Verification items for the finished model (mm, model axes). Face numbers are marked on the shaded views. A direction names the side the tool comes from. Round coordinates to 2 decimals unless told otherwise and drop trailing zeros. One line per item, written item: value. Start each with the question number.
from build123d import *

# Parameters (mm, degrees)
SKETCH1_R           = 8.345
SKETCH1_R_2         = 7.045
BOSS_EXTRUDE1_DEPTH = 7.92
SKETCH2_R           = 7.045000007
BOSS_EXTRUDE2_DEPTH = 1.02
BOSS_EXTRUDE3_REACH = 9.92
BOSS_EXTRUDE4_DEPTH = 0.51
SKETCH5_W           = 1.28
SKETCH5_H           = 2.28
SKETCH5_W_2         = 2.28
SKETCH5_H_2         = 1.28
BOSS_EXTRUDE5_DEPTH = 2.41
CUT_EXTRUDE1_DEPTH  = 9.985
CUT_EXTRUDE2_DEPTH  = 2.41
CUT_EXTRUDE3_DEPTH  = 2.41


with BuildPart() as part:
    # Sketch1 → Boss-Extrude1 (new body)
    with BuildSketch(Plane(origin=(0, 0, 0), x_dir=(1, 0, 0), z_dir=(0, 1, 0))):
        Circle(SKETCH1_R)
        Circle(SKETCH1_R_2, mode=Mode.SUBTRACT)
    extrude(amount=BOSS_EXTRUDE1_DEPTH)

    # Sketch2 → Boss-Extrude2 (add)
    with BuildSketch(Plane(origin=(0, 0, 0), x_dir=(1, 0, 0), z_dir=(0, 1, 0))):
        Circle(SKETCH2_R)
    extrude(amount=BOSS_EXTRUDE2_DEPTH)

    # Sketch3 → Boss-Extrude3 (add, up to next)
    with BuildSketch(Plane(origin=(0, 7.92, 0), x_dir=(1, 0, 0), z_dir=(0, 1, 0)), mode=Mode.PRIVATE) as boss_extrude3_sk1:
        with BuildLine():
            Line((-0.455000106, 4.724999874), (0.455000106, 4.724999874))
            Line((0.455000106, 4.724999874), (0.455000106, 8.332586627))
            ThreePointArc((0.455000106, 8.332586627), (0, 8.345), (-0.455000106, 8.332586627))
            Line((-0.455000106, 8.332586627), (-0.455000106, 4.724999874))
        make_face()
    boss_extrude3_tool1 = extrude(boss_extrude3_sk1.sketch, amount=-BOSS_EXTRUDE3_REACH, mode=Mode.PRIVATE) - part.part
    add(boss_extrude3_tool1.solids().sort_by_distance((0, 7.92, -6.532934))[0])
    # Sketch3 → Boss-Extrude3 (add, up to next)
    with BuildSketch(Plane(origin=(0, 7.92, 0), x_dir=(1, 0, 0), z_dir=(0, 1, 0)), mode=Mode.PRIVATE) as boss_extrude3_sk2:
        with BuildLine():
            Line((3.019345792, 3.662813112), (5.570294849, 6.213762169))
            ThreePointArc((5.570294849, 6.213762169), (5.900806089, 5.900806089), (6.213762169, 5.570294849))
            Line((6.213762169, 5.570294849), (3.662813112, 3.019345792))
            Line((3.662813112, 3.019345792), (3.019345792, 3.662813112))
        make_face()
    boss_extrude3_tool2 = extrude(boss_extrude3_sk2.sketch, amount=-BOSS_EXTRUDE3_REACH, mode=Mode.PRIVATE) - part.part
    add(boss_extrude3_tool2.solids().sort_by_distance((4.619482, 7.92, -4.619482))[0])
    # Sketch3 → Boss-Extrude3 (add, up to next)
    with BuildSketch(Plane(origin=(0, 7.92, 0), x_dir=(1, 0, 0), z_dir=(0, 1, 0)), mode=Mode.PRIVATE) as boss_extrude3_sk3:
        with BuildLine():
            Line((4.724999874, 0.455000106), (8.332586627, 0.455000106))
            ThreePointArc((8.332586627, 0.455000106), (8.345, 0), (8.332586627, -0.455000106))
            Line((8.332586627, -0.455000106), (4.724999874, -0.455000106))
            Line((4.724999874, -0.455000106), (4.724999874, 0.455000106))
        make_face()
    boss_extrude3_tool3 = extrude(boss_extrude3_sk3.sketch, amount=-BOSS_EXTRUDE3_REACH, mode=Mode.PRIVATE) - part.part
    add(boss_extrude3_tool3.solids().sort_by_distance((6.532934, 7.92, 0))[0])
    # Sketch3 → Boss-Extrude3 (add, up to next)
    with BuildSketch(Plane(origin=(0, 7.92, 0), x_dir=(1, 0, 0), z_dir=(0, 1, 0)), mode=Mode.PRIVATE) as boss_extrude3_sk4:
        with BuildLine():
            Line((3.662813112, -3.019345792), (6.213762169, -5.570294849))
            ThreePointArc((6.213762169, -5.570294849), (5.900806089, -5.900806089), (5.570294849, -6.213762169))
            Line((5.570294849, -6.213762169), (3.019345792, -3.662813112))
            Line((3.019345792, -3.662813112), (3.662813112, -3.019345792))
        make_face()
    boss_extrude3_tool4 = extrude(boss_extrude3_sk4.sketch, amount=-BOSS_EXTRUDE3_REACH, mode=Mode.PRIVATE) - part.part
    add(boss_extrude3_tool4.solids().sort_by_distance((4.619482, 7.92, 4.619482))[0])
    # Sketch3 → Boss-Extrude3 (add, up to next)
    with BuildSketch(Plane(origin=(0, 7.92, 0), x_dir=(1, 0, 0), z_dir=(0, 1, 0)), mode=Mode.PRIVATE) as boss_extrude3_sk5:
        with BuildLine():
            Line((0.455000106, -4.724999874), (0.455000106, -8.332586627))
            ThreePointArc((0.455000106, -8.332586627), (0, -8.345), (-0.455000106, -8.332586627))
            Line((-0.455000106, -8.332586627), (-0.455000106, -4.724999874))
            Line((-0.455000106, -4.724999874), (0.455000106, -4.724999874))
        make_face()
    boss_extrude3_tool5 = extrude(boss_extrude3_sk5.sketch, amount=-BOSS_EXTRUDE3_REACH, mode=Mode.PRIVATE) - part.part
    add(boss_extrude3_tool5.solids().sort_by_distance((0, 7.92, 6.532934))[0])
    # Sketch3 → Boss-Extrude3 (add, up to next)
    with BuildSketch(Plane(origin=(0, 7.92, 0), x_dir=(1, 0, 0), z_dir=(0, 1, 0)), mode=Mode.PRIVATE) as boss_extrude3_sk6:
        with BuildLine():
            Line((-3.019345792, -3.662813112), (-5.570294849, -6.213762169))
            ThreePointArc((-5.570294849, -6.213762169), (-5.900806089, -5.900806089), (-6.213762169, -5.570294849))
            Line((-6.213762169, -5.570294849), (-3.662813112, -3.019345792))
            Line((-3.662813112, -3.019345792), (-3.019345792, -3.662813112))
        make_face()
    boss_extrude3_tool6 = extrude(boss_extrude3_sk6.sketch, amount=-BOSS_EXTRUDE3_REACH, mode=Mode.PRIVATE) - part.part
    add(boss_extrude3_tool6.solids().sort_by_distance((-4.619482, 7.92, 4.619482))[0])
    # Sketch3 → Boss-Extrude3 (add, up to next)
    with BuildSketch(Plane(origin=(0, 7.92, 0), x_dir=(1, 0, 0), z_dir=(0, 1, 0)), mode=Mode.PRIVATE) as boss_extrude3_sk7:
        with BuildLine():
            Line((-4.724999874, -0.455000106), (-8.332586627, -0.455000106))
            ThreePointArc((-8.332586627, -0.455000106), (-8.345, 0), (-8.332586627, 0.455000106))
            Line((-8.332586627, 0.455000106), (-4.724999874, 0.455000106))
            Line((-4.724999874, 0.455000106), (-4.724999874, -0.455000106))
        make_face()
    boss_extrude3_tool7 = extrude(boss_extrude3_sk7.sketch, amount=-BOSS_EXTRUDE3_REACH, mode=Mode.PRIVATE) - part.part
    add(boss_extrude3_tool7.solids().sort_by_distance((-6.532934, 7.92, 0))[0])
    # Sketch3 → Boss-Extrude3 (add, up to next)
    with BuildSketch(Plane(origin=(0, 7.92, 0), x_dir=(1, 0, 0), z_dir=(0, 1, 0)), mode=Mode.PRIVATE) as boss_extrude3_sk8:
        with BuildLine():
            Line((-3.662813112, 3.019345792), (-6.213762169, 5.570294849))
            ThreePointArc((-6.213762169, 5.570294849), (-5.900806089, 5.900806089), (-5.570294849, 6.213762169))
            Line((-5.570294849, 6.213762169), (-3.019345792, 3.662813112))
            Line((-3.019345792, 3.662813112), (-3.662813112, 3.019345792))
        make_face()
    boss_extrude3_tool8 = extrude(boss_extrude3_sk8.sketch, amount=-BOSS_EXTRUDE3_REACH, mode=Mode.PRIVATE) - part.part
    add(boss_extrude3_tool8.solids().sort_by_distance((-4.619482, 7.92, -4.619482))[0])

    # Sketch4 → Boss-Extrude4 (add)
    with BuildSketch(Plane.XZ):
        with BuildLine():
            Line((-3.069700642, 2.308712987), (-6.179087875, 5.238791894))
            ThreePointArc((-6.179087875, 5.238791894), (-8.097423758, -0.240407921), (-5.857404636, -5.596148534))
            Line((-5.857404636, -5.596148534), (-2.927325729, -2.486761301))
            ThreePointArc((-2.927325729, -2.486761301), (-3.839300032, -0.113986642), (-3.069700642, 2.308712987))
        make_face()
        with BuildLine():
            Line((2.308712987, 3.069700642), (5.238791894, 6.179087875))
            ThreePointArc((5.238791894, 6.179087875), (-0.240407921, 8.097423758), (-5.596148534, 5.857404636))
            Line((-5.596148534, 5.857404636), (-2.486761301, 2.927325729))
            ThreePointArc((-2.486761301, 2.927325729), (-0.113986642, 3.839300032), (2.308712987, 3.069700642))
        make_face()
        with BuildLine():
            ThreePointArc((8.100991759, 0), (7.519203886, 3.014571346), (5.857404636, 5.596148534))
            Line((5.857404636, 5.596148534), (2.927325729, 2.486761301))
            ThreePointArc((2.927325729, 2.486761301), (3.605346841, 1.324647819), (3.840991759, 0))
            ThreePointArc((3.840991759, 0), (3.643069623, -1.217070832), (3.069700642, -2.308712987))
            Line((3.069700642, -2.308712987), (6.179087875, -5.238791894))
            ThreePointArc((6.179087875, -5.238791894), (7.605353622, -2.790101031), (8.100991759, 0))
        make_face()
        with BuildLine():
            ThreePointArc((-5.238791894, -6.179087875), (0.240407921, -8.097423758), (5.596148534, -5.857404636))
            Line((5.596148534, -5.857404636), (2.486761301, -2.927325729))
            ThreePointArc((2.486761301, -2.927325729), (0.113986642, -3.839300032), (-2.308712987, -3.069700642))
            Line((-2.308712987, -3.069700642), (-5.238791894, -6.179087875))
        make_face()
    extrude(amount=BOSS_EXTRUDE4_DEPTH)

    # Sketch5 → Boss-Extrude5 (add)
    with BuildSketch(Plane.XZ.offset(0.51)):
        with Locations((0, 4.98099181)):
            Rectangle(SKETCH5_W, SKETCH5_H)
        with Locations((4.98099181, 0)):
            Rectangle(SKETCH5_W_2, SKETCH5_H_2)
        with Locations((0, -4.98099181)):
            Rectangle(SKETCH5_W, SKETCH5_H)
        with Locations((-4.98099181, 0)):
            Rectangle(SKETCH5_W_2, SKETCH5_H_2)
    extrude(amount=BOSS_EXTRUDE5_DEPTH)

    # Sketch6 → Cut-Extrude1 (cut, through all)
    with BuildSketch(Plane(origin=(0, 0, -0.64), x_dir=(-1, 0, 0), z_dir=(0, 0, -1))):
        Polygon((6.12099181, -2.92), (3.84099181, -1.7), (3.84099181, -2.92), align=None)
    extrude(amount=-CUT_EXTRUDE1_DEPTH, mode=Mode.SUBTRACT)

    # Sketch7 → Cut-Extrude2 (cut)
    with BuildSketch(Plane(origin=(0.64, 0, 0), x_dir=(0, 0, -1), z_dir=(1, 0, 0))):
        Polygon((6.12099181, -2.92), (3.84099181, -1.7), (3.84099181, -2.92), align=None)
        Polygon((-6.12099181, -2.92), (-3.84099181, -2.92), (-3.84099181, -1.7), align=None)
    extrude(amount=-CUT_EXTRUDE2_DEPTH, mode=Mode.SUBTRACT)

    # Sketch6_3 → Cut-Extrude3 (cut)
    with BuildSketch(Plane(origin=(0, 0, -0.64), x_dir=(-1, 0, 0), z_dir=(0, 0, -1))):
        Polygon((-6.12099181, -2.92), (-3.84099181, -2.92), (-3.84099181, -1.7), align=None)
    extrude(amount=-CUT_EXTRUDE3_DEPTH, mode=Mode.SUBTRACT)


solid = part.part
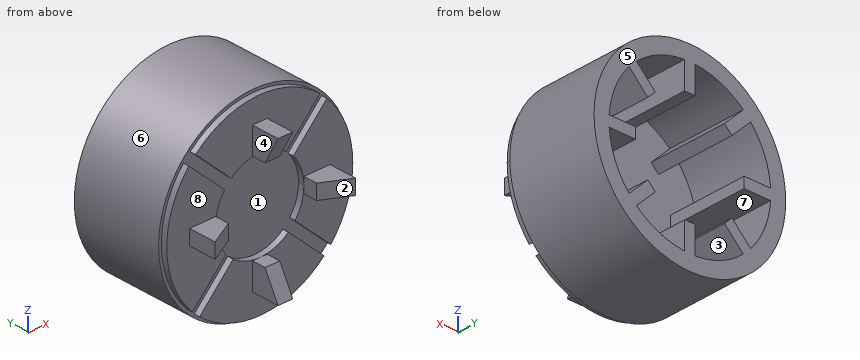
1. Depth check by flat-ended pin: pin 1 (0.7 mm diameter, centred on y = 6, z = -5.5, fed in from +X); pin 2 (1.4 mm diameter, centred on y = -1.5, z = 0, fed in from -X); pin 3 (1.1 mm diameter, centred on y = -1.5, z = -4.5, fed in from -X). Enter the tip coordinate at first touch or a pass-through.
2. Draft check along Z on the marked faces 6, 7 and 8. Enter one of: released by +Z, released by -Z, zero draft, split by the parting line, or undercut.
3. Scan lines: line 1 along X through (y, z) = (2, 0) (3 decimals); line 2 along X through (y, z) = (3.5, -4.5); line 3 along Z through (x, y) = (6.25, 3) (3 decimals). Record each from-to range of solid material in increasing order.
4. Tool access check on the marked faces 1, 2, 3, 4 and 5. Record the directions out of +Z, -Z, +X, -X, +Y, -Y that give a thin tool (end or side, any length) a straight path to the whole face; none if there is none.
Geometry check:
1. pin 1: stops at x = 6.57
1. pin 2: stops at x = -6.12
1. pin 3: stops at x = -0.64
2. face 6: split by the parting line
2. face 7: undercut
2. face 8: zero draft
3. line 1: x = -8.345 to -4.725, 4.725 to 8.345
3. line 2: x = -7.03 to -5.42, -5.14 to -3.86, 3.86 to 5.14, 5.42 to 7.03
3. line 3: z = -5.53 to -3.251, -0.455 to 0.455, 3.251 to 5.53
4. face 1: -Y
4. face 2: +Z, -Z, -Y
4. face 3: +Y
4. face 4: +Z, -Z, -X, -Y
4. face 5: +Z, -Z, +X, -X, +Y
